from build123d import *

# Parameters (mm, degrees)
SKETCH1_W                 = 40
SKETCH1_H                 = 40
BOSS_EXTRUDE1_DEPTH       = 7.5
F_4_40_TAPPED_HOLE1_D     = 2.2606
F_4_40_TAPPED_HOLE1_DEPTH = 7.6
F_4_40_TAPPED_HOLE1_TIP   = 0.679152758
F_4_40_TAPPED_HOLE2_D     = 2.2606
F_4_40_TAPPED_HOLE2_DEPTH = 7.6
F_4_40_TAPPED_HOLE2_TIP   = 0.679152758
F_4_40_TAPPED_HOLE3_D     = 2.2606
F_4_40_TAPPED_HOLE3_DEPTH = 7.6
F_4_40_TAPPED_HOLE3_TIP   = 0.679152758
F_4_40_TAPPED_HOLE4_D     = 2.2606
F_4_40_TAPPED_HOLE4_DEPTH = 7.6
F_4_40_TAPPED_HOLE4_TIP   = 0.679152758


with BuildPart() as part:
    # Sketch1 → Boss-Extrude1 (new body)
    with BuildSketch(Plane(origin=(0, 0, 0), x_dir=(1, 0, 0), z_dir=(0, 1, 0))):
        Rectangle(SKETCH1_W, SKETCH1_H)
    extrude(amount=BOSS_EXTRUDE1_DEPTH)

    # #4-40 Tapped Hole1
    with Locations(Plane.ZY.offset(20)):
        with Locations((-15, 3.75), (15, 3.75)):
            Hole(F_4_40_TAPPED_HOLE1_D / 2, depth=F_4_40_TAPPED_HOLE1_DEPTH)
            with Locations((0, 0, -(F_4_40_TAPPED_HOLE1_DEPTH + F_4_40_TAPPED_HOLE1_TIP / 2))):  # 118° drill point
                Cone(0, F_4_40_TAPPED_HOLE1_D / 2, F_4_40_TAPPED_HOLE1_TIP, mode=Mode.SUBTRACT)

    # #4-40 Tapped Hole2
    with Locations(Plane(origin=(20, 0, 0), x_dir=(0, 0, -1), z_dir=(1, 0, 0))):
        with Locations((-15, 3.75), (15, 3.75)):
            Hole(F_4_40_TAPPED_HOLE2_D / 2, depth=F_4_40_TAPPED_HOLE2_DEPTH)
            with Locations((0, 0, -(F_4_40_TAPPED_HOLE2_DEPTH + F_4_40_TAPPED_HOLE2_TIP / 2))):  # 118° drill point
                Cone(0, F_4_40_TAPPED_HOLE2_D / 2, F_4_40_TAPPED_HOLE2_TIP, mode=Mode.SUBTRACT)

    # #4-40 Tapped Hole3
    with Locations(Plane(origin=(0, 0, -20), x_dir=(-1, 0, 0), z_dir=(0, 0, -1))):
        with Locations((-10, 3.75), (10, 3.75)):
            Hole(F_4_40_TAPPED_HOLE3_D / 2, depth=F_4_40_TAPPED_HOLE3_DEPTH)
            with Locations((0, 0, -(F_4_40_TAPPED_HOLE3_DEPTH + F_4_40_TAPPED_HOLE3_TIP / 2))):  # 118° drill point
                Cone(0, F_4_40_TAPPED_HOLE3_D / 2, F_4_40_TAPPED_HOLE3_TIP, mode=Mode.SUBTRACT)

    # #4-40 Tapped Hole4
    with Locations(Plane.XY.offset(20)):
        with Locations((-10, 3.75), (10, 3.75)):
            Hole(F_4_40_TAPPED_HOLE4_D / 2, depth=F_4_40_TAPPED_HOLE4_DEPTH)
            with Locations((0, 0, -(F_4_40_TAPPED_HOLE4_DEPTH + F_4_40_TAPPED_HOLE4_TIP / 2))):  # 118° drill point
                Cone(0, F_4_40_TAPPED_HOLE4_D / 2, F_4_40_TAPPED_HOLE4_TIP, mode=Mode.SUBTRACT)


solid = part.part
Geometry: final body of the model. Coordinates: model frame, mm. A direction names the side the tool comes from. Coordinates: 2 decimals unless noted, no trailing zeros. Order: outer loops, then holes, each group sorted by start corner. A loop starts at its lowest first (then second) coordinate and runs counter-clockwise, first axis right, second up.
(1) Draft query along Y for faces 6 (the face through (0, 0, 0)), 7 (the face through (-10.091, 3.576, -11.839)), 8 (the face through (9.103, 3.062, -16.147)), 9 (the face through (0, 7.5, 0)). Return one class per face: pulls with the +Y half, pulls with the -Y half, needs draft (parallel to the pull), parting line crosses it, or undercut.
(2) Access query for faces 1 (the face through (-10.897, 3.062, -16.147)), 2 (the face through (-16.15, 3.8, 16.13)), 3 (the face through (10.897, 3.062, 16.147)), 4 (the face through (16.147, 3.062, 14.103)), 5 (the face through (0, 4, -20)). Directions: +Z, -Z, +X, -X, +Y, -Y. A direction counts if a zero-diameter tool reaches every point of the face in a straight line with its end or side. Return the directions, or none.
(3) First-contact query: pin 1 (1.8 mm diameter, centred on y = 3.75, z = 15, fed in from +X); pin 2 (2.5 mm diameter, centred on x = 10, y = 3.75, fed in from +Z); pin 3 (1.8 mm diameter, centred on x = 10, y = 3.75, fed in from -Z); pin 4 (1.4 mm diameter, centred on x = -10, y = 3.75, fed in from -Z). Flat tips, straight axial feed; report the tip coordinate or a pass-through.
(4) Material intervals for probe 1 along Z at (x, y) = (17, 3.75); probe 2 along X at (y, z) = (3.75, 16.5); probe 3 along X at (y, z) = (3, -15.5), sorted ascending.
(5) Section query A-A (x = 13.5). Return the cut outline in (y, z), plus the area to 3 significant figures.
Solution:
1. face 6: pulls with the -Y half
1. face 7: undercut
1. face 8: undercut
1. face 9: pulls with the +Y half
2. face 1: -Z
2. face 2: -X
2. face 3: +Z
2. face 4: +X
2. face 5: -Z, +X, -X, +Y, -Y
3. pin 1: stops at x = 12.26
3. pin 2: stops at z = 20
3. pin 3: stops at z = -12.26
3. pin 4: stops at z = -12.14
4. probe 1: z = -20 to -16.13, -13.87 to 13.87, 16.13 to 20
4. probe 2: x = -20 to -11.13, -8.87 to 8.87, 11.13 to 20
4. probe 3: x = -12.26 to -10.85, -9.15 to 9.15, 10.85 to 12.26
5. outline: (0, -20) - (7.5, -20) - (7.5, 20) - (0, 20) - close; hole circle Ø2.26 at (3.75, -15); hole circle Ø2.26 at (3.75, 15)
5. area: 292 mm2
